```python
from build123d import *

# Parameters (mm, degrees)
SKETCH_W      = 114
SKETCH_H      = 50
PAD_DEPTH     = 4
SKETCH001_R   = 11.25
SKETCH001_R_2 = 2.25
SKETCH001_R_3 = 1.75
POCKET_DEPTH  = 4.001
CHAMFER_SIZE  = 2
FILLET_R      = 5


with BuildPart() as part:
    # Sketch → Pad (new body)
    with BuildSketch(Plane.XY):
        Rectangle(SKETCH_W, SKETCH_H)
    extrude(amount=PAD_DEPTH)

    # Sketch001 → Pocket (cut, through all)
    with BuildSketch(Plane.XY.offset(4)):
        Circle(SKETCH001_R)
        with Locations((-47, 18)):
            Circle(SKETCH001_R_2)
        with Locations((-47, -18)):
            Circle(SKETCH001_R_2)
        with Locations((47, 18)):
            Circle(SKETCH001_R_2)
        with Locations((47, -18)):
            Circle(SKETCH001_R_2)
        with Locations((-9.899495, 9.899495)):
            Circle(SKETCH001_R_3)
        with Locations((9.899495, 9.899495)):
            Circle(SKETCH001_R_3)
        with Locations((9.899495, -9.899495)):
            Circle(SKETCH001_R_3)
        with Locations((-9.899495, -9.899495)):
            Circle(SKETCH001_R_3)
    extrude(amount=-POCKET_DEPTH, mode=Mode.SUBTRACT)

    # Chamfer
    chamfer_edges = [part.edges().sort_by_distance(p)[0] for p in [
        (0, -25, 0),
    ]]
    chamfer(chamfer_edges, length=CHAMFER_SIZE)

    # Fillet
    fillet_edges = [part.edges().sort_by_distance(p)[0] for p in [
        (-57, -25, 3),
        (-57, 25, 2),
        (57, -25, 3),
        (57, 25, 2),
    ]]
    fillet(fillet_edges, radius=FILLET_R)


solid = part.part
```
Design review of the part built by this model. Coordinates are the model's own, in mm. Coordinates: 2 decimals unless noted, no trailing zeros. Loops run counter-clockwise (first coordinate to the right, second up) from the corner with the lowest first, then second, coordinate; pieces in that order, holes last. Notation, with made-up numbers: M 0,-33.5 L 59,-33.5 A19 cw 59,-12.5 Z; hole C -38,48 d11. An arc over 180 degrees is marked long. One line per question, with ' | ' between items.
(1) We need section A-A (y = 18). Give the boundary of the cut face in (x, z).
Filled in:
outline: M -57,0 L -49.25,0 L -49.25,4 L -57,4 Z; M -44.75,0 L 44.75,0 L 44.75,4 L -44.75,4 Z; M 49.25,0 L 57,0 L 57,4 L 49.25,4 Z
(2) Wall thickness on probe 1 along Y at (x, z) = (-47, 2.1); probe 2 along Y at (x, z) = (46, 2.4); probe 3 along Y at (x, z) = (10, 1.25): over which ranges is each line inside the solid? List them lowest first.
Filled in:
probe 1: y = -25 to -20.25, -15.75 to 15.75, 20.25 to 25 | probe 2: y = -25 to -20.02, -15.98 to 15.98, 20.02 to 25 | probe 3: y = -24.25 to -11.65, -8.15 to -5.15, 5.15 to 8.15, 11.65 to 25
(3) Draft analysis for pull direction X (two halves, no side actions). For faces 1 (the face through (11.516, 9.229, 2.028)), 2 (the face through (55, 24, 2)), 3 (the face through (-1, 25, 2)), state which applies: released by +X, released by -X, zero draft, split by the parting line, or undercut.
Filled in:
face 1: undercut | face 2: released by +X | face 3: zero draft
(4) We need section B-B (x = 0). Give the boundary of the cut face in (y, z).
Filled in:
outline: M -25,2 L -23,0 L -11.25,0 L -11.25,4 L -25,4 Z; M 11.25,0 L 25,0 L 25,4 L 11.25,4 Z
(5) We need section C-C (y = 2). Give the boundary of the cut face in (x, z).
Filled in:
outline: M -57,0 L -11.07,0 L -11.07,4 L -57,4 Z; M 11.07,0 L 57,0 L 57,4 L 11.07,4 Z
(6) We need section D-D (z = 0.95). Count the separate pieces of the cut face and the enclosed holes in it, and give its area (3 significant figures).
Filled in:
separate pieces: 1 | enclosed holes: 9 | area: 5,070 mm^2
